Work out the finished part from the listing and answer in its coordinate system (mm). A direction names the side the tool comes from. Round coordinates to 2 decimals unless told otherwise and drop trailing zeros. Order: outer loops, then holes, each group sorted by start corner. A loop starts at its lowest first (then second) coordinate and runs counter-clockwise, first axis right, second up. Notation, with made-up numbers: M -13,55.25 L 44,55.25 A31 ccw 44,81.25 Z; hole C -4,-25.75 d5. An arc over 180 degrees is marked long. Return JSON: item names as keys, results as strings.
from build123d import *

# Parameters (mm, degrees)
SKETCH1_W           = 200
SKETCH1_H           = 175
BOSS_EXTRUDE1_DEPTH = 50
BOSS_EXTRUDE2_DEPTH = 175
SKETCH4_W           = 200
SKETCH4_H           = 10
BOSS_EXTRUDE3_DEPTH = 50
SKETCH6_W           = 200
SKETCH6_H           = 10
BOSS_EXTRUDE4_DEPTH = 50


with BuildPart() as part:
    # Sketch1 → Boss-Extrude1 (new body)
    with BuildSketch(Plane(origin=(0, 0, 0), x_dir=(1, 0, 0), z_dir=(0, 1, 0))):
        with Locations((0, 14.608639935)):
            Rectangle(SKETCH1_W, SKETCH1_H)
    extrude(amount=BOSS_EXTRUDE1_DEPTH)

    # Sketch3 → Boss-Extrude2 (add)
    with BuildSketch(Plane.XY.offset(72.891360065)):
        Polygon((-80, 50), (0, 125), (80, 50), align=None)
    extrude(amount=-BOSS_EXTRUDE2_DEPTH)

    # Sketch4 → Boss-Extrude3 (add)
    with BuildSketch(Plane(origin=(0, 50, 0), x_dir=(1, 0, 0), z_dir=(0, 1, 0))):
        with Locations((0, 54.608639935)):
            Rectangle(SKETCH4_W, SKETCH4_H)
    extrude(amount=BOSS_EXTRUDE3_DEPTH)

    # Sketch6 → Boss-Extrude4 (add)
    with BuildSketch(Plane(origin=(0, 50, 0), x_dir=(1, 0, 0), z_dir=(0, 1, 0))):
        with Locations((0, -25.391360065)):
            Rectangle(SKETCH6_W, SKETCH6_H)
    extrude(amount=BOSS_EXTRUDE4_DEPTH)


solid = part.part
Item 1: Find section A-A (x = 56). Determine the outline of the cut face in (y, z).
Output:
{"outline": "M 0,-102.11 L 72.5,-102.11 L 72.5,-59.61 L 100,-59.61 L 100,-49.61 L 72.5,-49.61 L 72.5,20.39 L 100,20.39 L 100,30.39 L 72.5,30.39 L 72.5,72.89 L 0,72.89 Z"}
Item 2: The mould has two halves that part along Z. Classify faces 1 (the flat face through (-72, 80, 30.391)), 2 (the flat face through (71, 80, -59.609)), 3 (the flat face through (90, 50, -15)), 4 (the flat face through (63, 100, -55)): pulls with the +Z half, pulls with the -Z half, needs draft (parallel to the pull), parting line crosses it, or undercut.
Output:
{"face 1": "pulls with the +Z half", "face 2": "pulls with the -Z half", "face 3": "undercut", "face 4": "needs draft"}
Item 3: Which of the six approach directions +Z, -Z, +X, -X, +Y, -Y give full straight-line access (tool end or side, diameter ignored) to faces 5 (the flat face through (-90, 50, 51)), 6 (the flat face through (-72, 80, -49.609)), 7 (the flat face through (63, 100, 25))?
Output:
{"face 5": "+Z, -X, +Y", "face 6": "-X, +Y", "face 7": "+Z, -Z, +X, +Y"}
Item 4: Find section B-B (z = -77.5). Determine the outline of the cut face in (x, y), plus the area to 3 significant figures.
Output:
{"outline": "M -100,0 L 100,0 L 100,50 L 80,50 L 0,125 L -80,50 L -100,50 Z", "area": "16,000 mm^2"}
Item 5: Each of these flat-tipped pins is pushed along its axis until it touches: pin 1 (22 mm diameter, centred on x = -87.5, z = 55, fed in from +Y); pin 2 (15 mm diameter, centred on x = -75.5, y = 78, fed in from -Z); pin 3 (15 mm diameter, centred on x = 57, y = 72, fed in from -Z); pin 4 (8 mm diameter, centred on x = 74.5, z = 26, fed in from +Y). Where does it stop, or does it pass through?
Output:
{"pin 1": "stops at y = 53.28", "pin 2": "stops at z = -59.61", "pin 3": "stops at z = -102.11", "pin 4": "stops at y = 100"}
Item 6: Find section C-C (y = 64). Determine the outline of the cut face in (x, z), plus the area to 3 significant figures.
Output:
{"outline": "M -100,-59.61 L -65.07,-59.61 L -65.07,-102.11 L 65.07,-102.11 L 65.07,-59.61 L 100,-59.61 L 100,-49.61 L 65.07,-49.61 L 65.07,20.39 L 100,20.39 L 100,30.39 L 65.07,30.39 L 65.07,72.89 L -65.07,72.89 L -65.07,30.39 L -100,30.39 L -100,20.39 L -65.07,20.39 L -65.07,-49.61 L -100,-49.61 Z", "area": "24,200 mm^2"}
Item 7: Consider line 1 along Y through (x, z) = (-46, 20.5); line 2 along Y through (x, z) = (-48, -3.5); line 3 along X through (y, z) = (67.5, 40). Determine where each line is inside the solid, lowest interval first. Write a range as [from, to].
Output:
{"line 1": "y = [0, 100]", "line 2": "y = [0, 80]", "line 3": "x = [-61.33, 61.33]"}
Item 8: Find section D-D (x = -38). Determine the outline of the cut face in (y, z) (3 decimals), plus the area to 3 significant figures.
Output:
{"outline": "M 0,-102.109 L 89.375,-102.109 L 89.375,-59.609 L 100,-59.609 L 100,-49.609 L 89.375,-49.609 L 89.375,20.391 L 100,20.391 L 100,30.391 L 89.375,30.391 L 89.375,72.891 L 0,72.891 Z", "area": "15,900 mm^2"}
